Print and shaded views of the part. All mm, measured from the part's lowest x, y and z. Give positions to 0.01 mm unless a question says otherwise; leave off trailing zeros. Loops run counter-clockwise (first coordinate to the right, second up) from the corner with the lowest first, then second, coordinate; pieces in that order, holes last. Notation, with made-up numbers: M 41,-30 L 58,-30 A22 ccw 58,-5 Z; hole C -19.75,12 d1. An arc over 180 degrees is marked long. Answer as CSV lines item,"result".
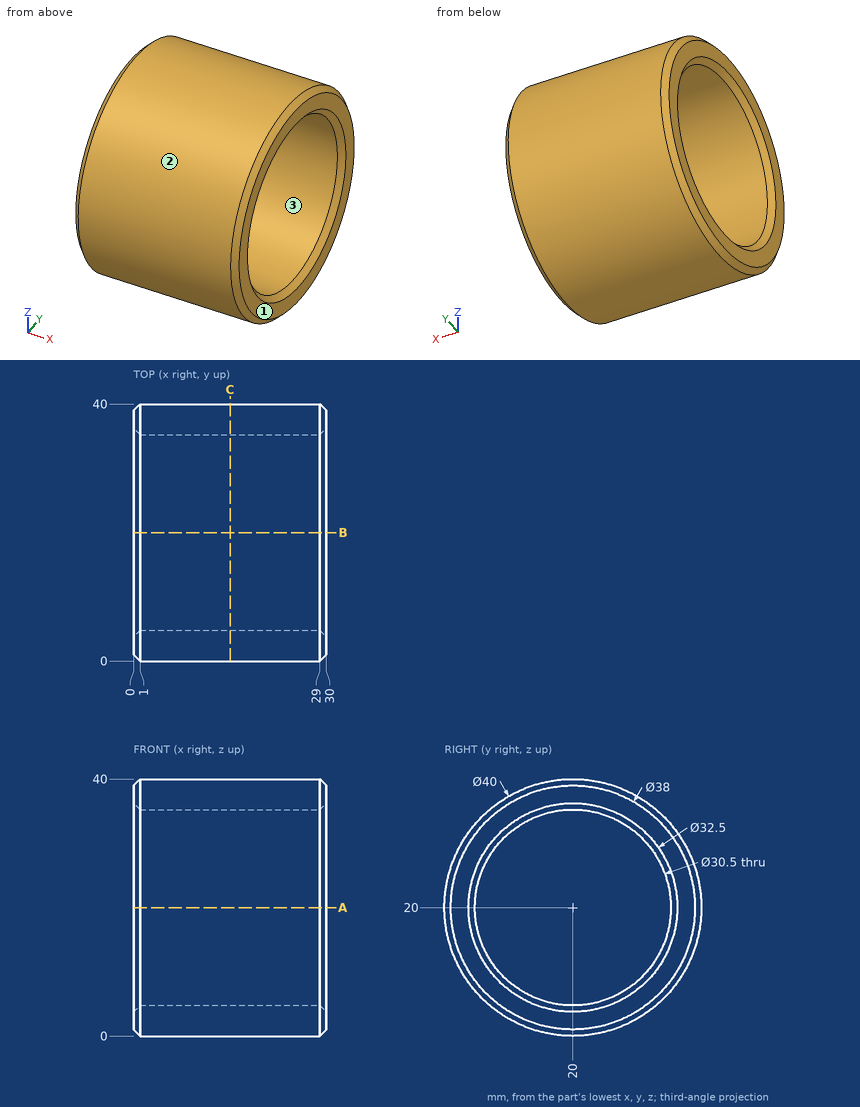
Q1. Wall check: line 1 (Y direction, x = 15.5, z = 20); line 2 (Z direction, x = 19.75, y = 8.5); line 3 (Y direction, x = 7, z = 8). Give the ranges that are in metal, low to high. Write a range as [from, to].
Solution:
line 1,"y = [0, 4.75], [35.25, 40]"
line 2,"z = [3.64, 9.98], [30.02, 36.36]"
line 3,"y = [4, 10.59], [29.41, 36]"
Q2. Mould opens along Y. For the marked faces 1, 2 and 3 say: released by +Y, released by -Y, zero draft, split by the parting line, or undercut.
Solution:
face 1,"zero draft"
face 2,"split by the parting line"
face 3,"undercut"
Q3. Pin check, flat tips, straight feed: P1, Ø3, axis at x = 22, z = 5.5, coming from the +Y side; P2, Ø3, axis at x = 16.5, z = 22, coming from the +Y side; P3, Ø3, axis at x = 17, y = 24, coming from the +Z side. Stop position of each tip, or through.
Solution:
P1,"stops at y = 35.2"
P2,"stops at y = 39.99"
P3,"stops at z = 39.84"
Q4. Cut at C-C (x = 15). Write the cut outline in (y, z).
Solution:
outline,"C 20,20 d40; hole C 20,20 d30.5"
Q5. Cut at A-A (z = 20). Write the cut outline in (x, y).
Solution:
outline,"M 0,1 L 1,0 L 29,0 L 30,1 L 30,3.75 L 29,4.75 L 1,4.75 L 0,3.75 Z; M 0,36.25 L 1,35.25 L 29,35.25 L 30,36.25 L 30,39 L 29,40 L 1,40 L 0,39 Z"
